Autodesk Inventor part; units mm, degrees
ref_plane "Plano inicial" through (0, 0, 0) normal (0, 0, 1) x (1, 0, 0)
ref_plane "Plano final" through (0, 0, 2190) normal (0, 0, 1) x (1, 0, 0)
ref_plane "YZ Plane" through (0, 0, 0) normal (1, 0, 0) x (0, 1, 0)
ref_plane "Plano inicial" through (0, 0, 0) normal (0, 0, 1) x (1, 0, 0)
ref_plane "Plano final" through (0, 0, 2190) normal (0, 0, 1) x (1, 0, 0)
sketch "Boceto" plane through (0, 0, 0) normal (0, 0, 1) x (1, 0, 0)
  line L0 (-25.4, -19.05) -> (-25.4, 19.05)
  line L1 (-19.05, 25.4) -> (19.05, 25.4)
  line L2 (25.4, 19.05) -> (25.4, -19.05)
  line L3 (19.05, -25.4) -> (-19.05, -25.4)
  arc A0 (-25.4, -19.05) -> (-19.05, -25.4) centre (-19.05, -19.05) ccw
  arc A1 (-19.05, 25.4) -> (-25.4, 19.05) centre (-19.05, 19.05) ccw
  arc A2 (25.4, 19.05) -> (19.05, 25.4) centre (19.05, 19.05) ccw
  arc A3 (19.05, -25.4) -> (25.4, -19.05) centre (19.05, -19.05) ccw
  arc A4 (-19.05, 22.225) -> (-22.225, 19.05) centre (-19.05, 19.05) ccw
  line L4 (-19.05, 22.225) -> (19.05, 22.225)
  arc A5 (22.225, 19.05) -> (19.05, 22.225) centre (19.05, 19.05) ccw
  line L5 (22.225, 19.05) -> (22.225, -19.05)
  arc A6 (19.05, -22.225) -> (22.225, -19.05) centre (19.05, -19.05) ccw
  line L6 (19.05, -22.225) -> (-19.05, -22.225)
  arc A7 (-22.225, -19.05) -> (-19.05, -22.225) centre (-19.05, -19.05) ccw
  line L7 (-22.225, -19.05) -> (-22.225, 19.05)
  line L8 (0, 37.4012) -> (0, -37.4012) construction
  line L9 (-37.4012, 0) -> (37.4012, 0) construction
  dimension "d10" = 50.8
  dimension "d11" = 50.8
  dimension "d12" = 3.175
  dimension "d15" = 25.4
  dimension "d16" = 25.4
  dimension "d17" = 6.35
extrude "Cuerpo" add sketch "Boceto" along normal up to surface (2190 mm away) from surface at 0
sketch "Sketch3" plane through (0, 0, 0) normal (0, 0, 1) x (1, 0, 0)
  line L0 (0, 0) -> (10, 0)
ref_plane "Work Plane3" through (0, 0, 0) normal (0, -1, 0) x (1, 0, 0)
sketch "Boceto5" plane through (19.05, 25.4, 2190) normal (0, 1, 0) x (1, 0, 0)
  line L0 (-19.05, 2190) -> (-19.05, 0)
  line L1 (-38.1, 2190) -> (-38.1, 0)
  circle A0 centre (-19.05, 2094.8516) radius 9.017
  circle A1 centre (-19.05, 1326.4) radius 9.017
  circle A2 centre (-19.05, 539) radius 9.017
  line L2 (-38.1, 2190) -> (0, 2190)
  point P0 (-19.05, 2190)
  point P1 (-19.05, 2190)
  point P2 (-19.05, 2190)
  dimension "d20" = 18.034
  dimension "d21" = 18.034
  dimension "d22" = 18.034
  dimension "d23" = 1651
  dimension "d24" = 863.6
  dimension "d25" = 95.1484
extrude "Extrusión2" cut sketch "Boceto5" against normal blind 19.05
sketch "Sketch4" plane through (0, 0, 0) normal (0, -1, 0) x (1, 0, 0)
  line L0 (-2, 0) -> (12, 0)
  line L1 (-2, 2190) -> (12, 2190)
  dimension "d19" = 2190
equation "\"d10\" = G_H"
equation "\"d11\" = G_W"
equation "\"d12\" = G_T"
equation "\"d15\" = 0.5 * d10"
equation "\"d16\" = 0.5 * d11"
equation "\"d17\" = G_IR"
equation "\"d3\" = G_L"
equation "\"G_W\" = 50.8"
equation "\"G_H\" = 50.8"
equation "\"G_T\" = 3.175"
equation "\"G_IR\" = 6.35"
equation "\"G_L\" = d19"
equation "\"G_OFFSET_START\" = 0"
equation "\"G_OFFSET_END\" = 0"
equation "\"d14\" = G_OFFSET_END + B_L"
equation "\"B_L\" = 2190"
properties part number "AISC - 2 x 2 x 1/8 - 86,22" material "Acero, suave"
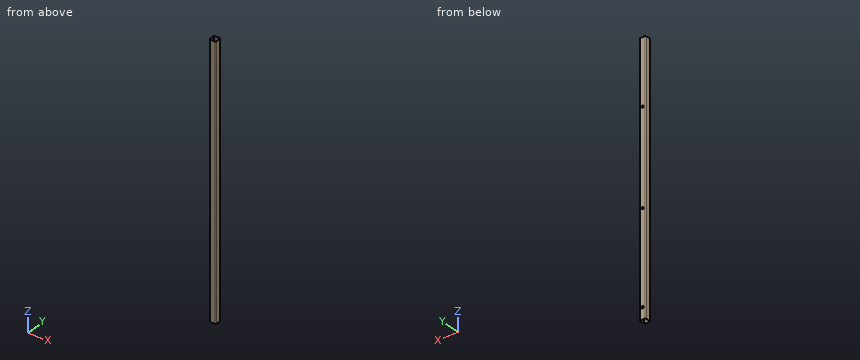
The model under review builds one solid part; all positions refer to its coordinate system, in mm. Give positions to 0.01 mm unless a question says otherwise; leave off trailing zeros. Order: outer loops, then holes, each group sorted by start corner. A loop starts at its lowest first (then second) coordinate and runs counter-clockwise, first axis right, second up. Notation, with made-up numbers: M -5.75,83.5 L 37.25,83.5 A34 ccw 37.25,121.5 Z; hole C 52.25,-23.75 d10. An arc over 180 degrees is marked long. Use one line per item in the form item = value. Start each with the question number.
Item 1: Insertion check: pin 1 Ø23.5 at (x, z) = (0, 95.15) entering from +Y. The pin has a flat end and moves straight along its axis. Give the tip position at first contact, or say it passes through.
Item 2: We need section B-B on z = 145.5. Give the boundary of the cut face in (x, y) (3 decimals).
Item 3: We need section A-A on x = 0. Give the boundary of the cut face in (y, z) (3 decimals), plus the area to 3 significant figures.
Item 4: To check wall thickness, follow line 1 along Z through (x, y) = (0, 23.45); line 2 along X through (y, z) = (-14, 1318.5) (3 decimals); line 3 along X through (y, z) = (24.7, 1651). State the ranges of each line that lie inside material, in increasing order. Write a range as from..to.
Completed:
q1.pin_1 = 25.4
q2.outline = M -25.4,-19.05 A6.35 ccw -19.05,-25.4 L 19.05,-25.4 A6.35 ccw 25.4,-19.05 L 25.4,19.05 A6.35 ccw 19.05,25.4 L -19.05,25.4 A6.35 ccw -25.4,19.05 Z; hole M -22.225,-19.05 A3.175 ccw -19.05,-22.225 L 19.05,-22.225 A3.175 ccw 22.225,-19.05 L 22.225,19.05 A3.175 ccw 19.05,22.225 L -19.05,22.225 A3.175 ccw -22.225,19.05 Z
q3.outline = M -25.4,0 L -22.225,0 L -22.225,2190 L -25.4,2190 Z; M 22.225,0 L 25.4,0 L 25.4,86.131 L 22.225,86.131 Z; M 22.225,104.165 L 25.4,104.165 L 25.4,854.583 L 22.225,854.583 Z; M 22.225,872.617 L 25.4,872.617 L 25.4,1641.983 L 22.225,1641.983 Z; M 22.225,1660.017 L 25.4,1660.017 L 25.4,2190 L 22.225,2190 Z
q3.area = 13,700 mm²
q4.line_1 = 0..86.13, 104.17..854.58, 872.62..1641.98, 1660.02..2190
q4.line_2 = -25.4..-22.225, 22.225..25.4
q4.line_3 = -21.95..-9.02, 9.02..21.95
